Geometry check sheet. Reference: the model listing, model coordinates, mm. A direction names the side the tool comes from. Round coordinates to 2 decimals unless told otherwise and drop trailing zeros. Write each loop counter-clockwise with the first axis right and the second up, starting at its lowest first coordinate (ties: lowest second). Pieces come first, ordered by that corner, then holes. Notation, with made-up numbers: M 67.25,-38 L 77.25,-38 A22 ccw 77.25,-32 Z; hole C 78.25,24.25 d7. An arc over 180 degrees is marked long. Answer in a Markdown table with one row per item. Add a question column.
from build123d import *

# Parameters (mm, degrees)
SKETCH1_R           = 2.1
SKETCH1_R_2         = 7
BOSS_EXTRUDE1_DEPTH = 10
FILLET1_R           = 2
SKETCH2_R           = 16.1
CUT_EXTRUDE1_DEPTH  = 8


with BuildPart() as part:
    # Sketch1 → Boss-Extrude1 (new body)
    with BuildSketch(Plane(origin=(0, 0, 0), x_dir=(1, 0, 0), z_dir=(0, 1, 0))):
        with BuildLine():
            Line((0, 18.1), (45, 18.1))
            ThreePointArc((45, 18.1), (67.641132128, 7.472867216), (73.932044859, -16.734182011))
            ThreePointArc((73.932044859, -16.734182011), (69.265817989, -19.932044859), (66.067955141, -15.265817989))
            ThreePointArc((66.067955141, -15.265817989), (61.486990751, 2.361454112), (45, 10.1))
            Line((45, 10.1), (10.576879596, -14.68807741))
            ThreePointArc((10.576879596, -14.68807741), (-17.225913635, -5.556788591), (0, 18.1))
        make_face()
        with Locations(Location((-8, 8, 0), (0, 0, 270))):
            Circle(SKETCH1_R, mode=Mode.SUBTRACT)
        with Locations(Location((8, 8, 0), (0, 0, 270))):
            Circle(SKETCH1_R, mode=Mode.SUBTRACT)
        with Locations(Location((8, -8, 0), (0, 0, 270))):
            Circle(SKETCH1_R, mode=Mode.SUBTRACT)
        with Locations(Location((-8, -8, 0), (0, 0, 270))):
            Circle(SKETCH1_R, mode=Mode.SUBTRACT)
        with Locations(Location((0, 0, 0), (0, 0, 270))):
            Circle(SKETCH1_R_2, mode=Mode.SUBTRACT)
        with BuildLine():
            Line((15.019986684, 10.1), (34.732321427, 10.1))
            Line((34.732321427, 10.1), (17.994323759, -1.953026484))
            ThreePointArc((17.994323759, -1.953026484), (17.572849381, 4.336469143), (15.019986684, 10.1))
        make_face(mode=Mode.SUBTRACT)
    extrude(amount=BOSS_EXTRUDE1_DEPTH)

    # Fillet1
    fillet1_edges = [part.edges().sort_by_distance(p)[0] for p in [
        (45, 5, -10.1),
        (15.019986684, 5, -10.1),
        (17.994323759, 5, 1.953026484),
        (34.732321427, 5, -10.1),
    ]]
    fillet(fillet1_edges, radius=FILLET1_R)

    # Sketch2 → Cut-Extrude1 (cut)
    with BuildSketch(Plane.XZ):
        with Locations(Location((0, 0, 0), (0, 0, 270))):
            Circle(SKETCH2_R)
    extrude(amount=-CUT_EXTRUDE1_DEPTH, mode=Mode.SUBTRACT)


solid = part.part
Item 1: Access from +Z, -Z, +X, -X, +Y, -Y to the whole of each face (thin tool, end or side, straight path). Record for faces 1 (the flat face through (23, 5, -10.1)), 2 (the cylindrical face through (-6.17, 3.94, -14.87)), 3 (the flat face through (29, 10, -4)).
Item 2: Section check C-C, the plane z = 8.5. Record the boundary of the cut face in (x, y).
Item 3: Gauge pin test, flat ends, axial feed: pin 1 Ø6 at (y, z) = (4, -5.5) entering from -X; pin 2 Ø9.5 at (x, z) = (5.5, -6) entering from -Y; pin 3 Ø3 at (x, y) = (6.5, 8.5) entering from +Z; pin 4 Ø5 at (x, z) = (34, -9) entering from -Y. Record the tip position at first contact, or that the pin passes through.
Item 4: Mould release check, pull along Z, two halves, no side actions. Record for faces 4 (the flat face through (35, 0, -5)), 5 (the cylindrical face through (-17.073, 4.93, 6.009)), 6 (the flat face through (22, 5, -18.1)), 7 (the flat face through (25.5, 4.93, -3.45)): +Z half, -Z half, draft (parallel to the pull), parting line (faces both ways), or undercut.
Item 5: Scan lines: probe 1 along Z at (x, y) = (-8, 9); probe 2 along Z at (x, y) = (8, 9.1); probe 3 along X at (y, z) = (9.1, 8). Record each from-to range of solid material in increasing order. Write a range as from..to.
Item 6: Section check A-A, the plane x = 27. Record the boundary of the cut face in (y, z), and give its area (3 significant figures).
Item 7: Section check B-B, the plane y = 1.5. Record the boundary of the cut face in (x, z), and give its area (3 significant figures).
Item 8: Section check D-D, the plane x = 8. Record the boundary of the cut face in (y, z), and give its area (3 significant figures).
Result sheet:
| question | item | result |
|---|---|---|
| 1 | face 1 | +Y, -Y |
| 1 | face 2 | -Y |
| 1 | face 3 | +Z, -Z, +X, -X, +Y |
| 2 | outline | M -15.98,0 L -13.67,0 L -13.67,8 L -10.04,8 L -10.04,10 L -15.98,10 Z; M -5.96,8 L 5.96,8 L 5.96,10 L -5.96,10 Z; M 10.04,8 L 13.67,8 L 13.67,0 L 19.17,0 L 19.17,10 L 10.04,10 Z; M 66.24,0 L 74.3,0 L 74.3,10 L 66.24,10 Z |
| 3 | pin 1 | stops at x = -17.93 |
| 3 | pin 2 | stops at y = 8 |
| 3 | pin 3 | stops at z = 17.4 |
| 3 | pin 4 | stops at y = 0 |
| 4 | face 4 | draft |
| 4 | face 5 | parting line |
| 4 | face 6 | -Z half |
| 4 | face 7 | undercut |
| 5 | probe 1 | z = -16.24..-10.1, -5.9..5.9, 10.1..16.24 |
| 5 | probe 2 | z = -18.1..-10.1, -5.9..5.9, 10.1..16.24 |
| 5 | probe 3 | x = -16.24..-10.1, -5.9..5.9, 10.1..19.86, 66.17..74.24 |
| 6 | outline | M 0,-18.1 L 10,-18.1 L 10,-10.1 L 0,-10.1 Z; M 0,-4.53 L 10,-4.53 L 10,2.86 L 0,2.86 Z |
| 6 | area | 154 mm^2 |
| 7 | outline | M 0,-18.1 L 45,-18.1 A29.43 ccw 73.93,16.73 A4 ccw 66.07,15.27 A21.43 cw 45.7,-10.09 A2 cw 44.46,-9.71 L 10.58,14.69 A18.1 ccw long Z; hole C 0,0 d32.2; hole M 16.57,-7.29 A2 ccw 18.4,-10.1 L 28.53,-10.1 A2 ccw 29.7,-6.48 L 21.17,-0.34 A2 ccw 18.01,-1.76 A18.1 cw Z |
| 7 | area | 1,060 mm^2 |
| 8 | outline | M 0,-18.1 L 10,-18.1 L 10,-10.1 L 8,-10.1 L 8,-13.97 L 0,-13.97 Z; M 0,13.97 L 8,13.97 L 8,10.1 L 10,10.1 L 10,16.24 L 0,16.24 Z; M 8,-5.9 L 10,-5.9 L 10,5.9 L 8,5.9 Z |
| 8 | area | 103 mm^2 |
